Check sheet for the drawn part. Datum: minimum x, y, z corner. Units: mm. Coordinates: 2 decimals unless noted, no trailing zeros. Order: outer loops, then holes, each group sorted by start corner. A loop starts at its lowest first (then second) coordinate and runs counter-clockwise, first axis right, second up. Notation, with made-up numbers: (28, 81.25) - (58, 81.25) arc R20 cw to (58, 105.25) - close; hole circle Ø4 at (-6, -37). An arc over 180 degrees is marked (long way). One line per item, written item: value. Start each with the question number.
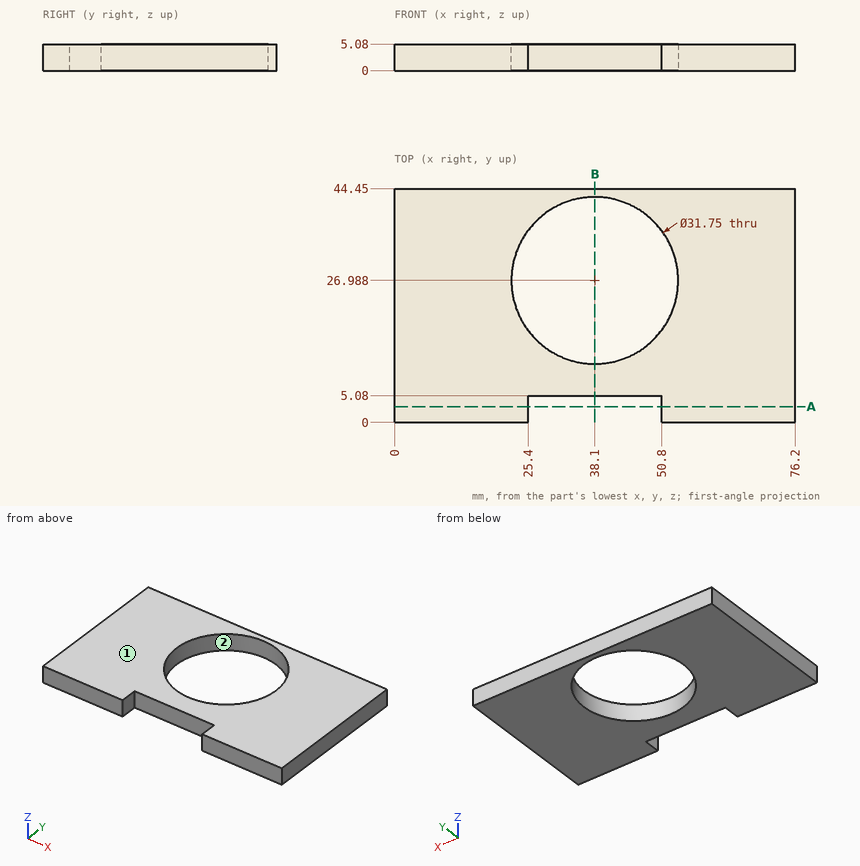
Q1. Cross-section at B-B, the plane x = 38.1. Enter the section's corners in (y, z), and give its area (3 significant figures).
Q2. Release check for a two-part mould opening along X. For the marked faces 1 and 2 record: released by +X, released by -X, zero draft, split by the parting line, or undercut.
Q3. Cross-section at A-A, the plane y = 3. Enter the section's corners in (x, z).
Q4. Gauge pin test, flat ends, axial feed: P1, Ø2, axis at x = 53.5, y = 9, coming from the -Z side; P2, Ø1, axis at x = 34, z = 1.5, coming from the -Y side. Record the tip position at first contact, or that the pin passes through.
Q5. Material ranges on probe 1 along Y at (x, z) = (38.1, 1.85); probe 2 along X at (y, z) = (2, 0.35); probe 3 along X at (y, z) = (18, 2.55) (1 decimal), recorded low to high.
Check result:
1. outline: (5.08, 0) - (11.11, 0) - (11.11, 5.08) - (5.08, 5.08) - close; (42.86, 0) - (44.45, 0) - (44.45, 5.08) - (42.86, 5.08) - close
1. area: 38.7 mm2
2. face 1: zero draft
2. face 2: undercut
3. outline: (0, 0) - (25.4, 0) - (25.4, 5.08) - (0, 5.08) - close; (50.8, 0) - (76.2, 0) - (76.2, 5.08) - (50.8, 5.08) - close
4. P1: stops at z = 0
4. P2: stops at y = 5.08
5. probe 1: y = 5.08 to 11.11, 42.86 to 44.45
5. probe 2: x = 0 to 25.4, 50.8 to 76.2
5. probe 3: x = 0 to 25, 51.2 to 76.2
